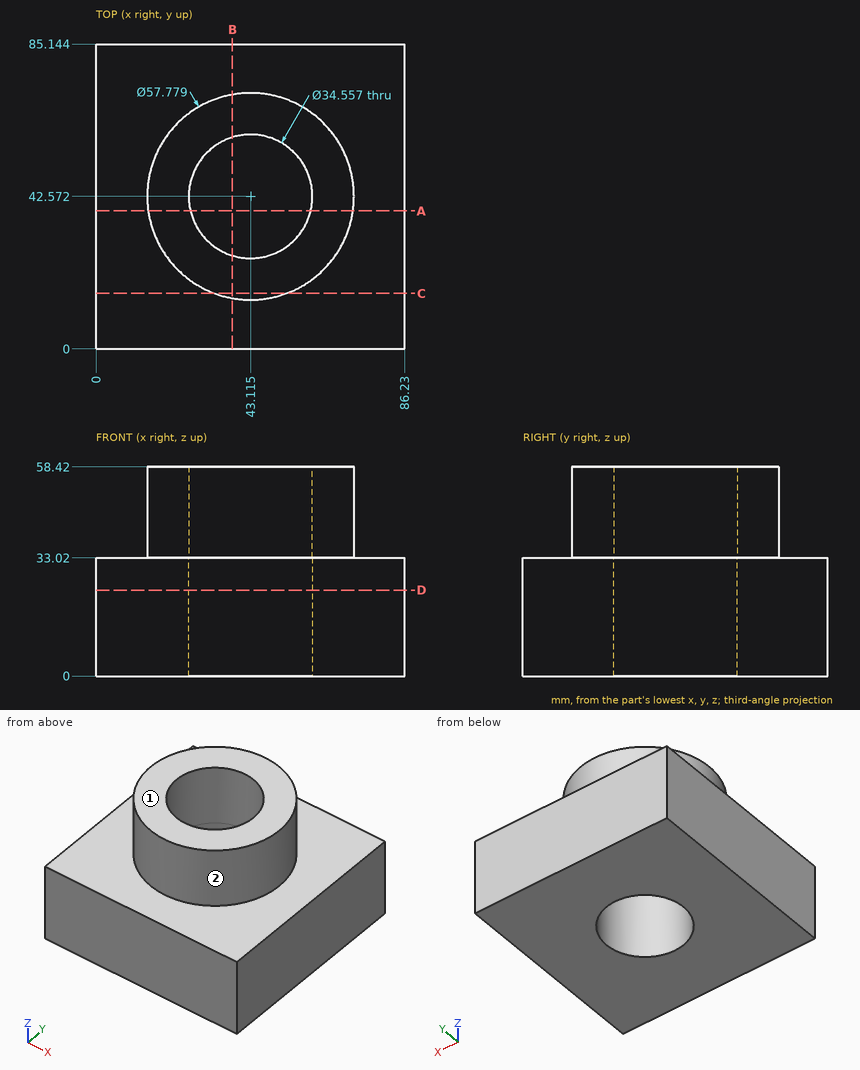
Geometry check sheet. Reference: drawing and pictorial views, mm from the part's lowest x, y, z. A direction names the side the tool comes from. Coordinates: 2 decimals unless noted, no trailing zeros. Order: outer loops, then holes, each group sorted by start corner. A loop starts at its lowest first (then second) coordinate and runs counter-clockwise, first axis right, second up.
1. Sectioned sample at A-A, the plane y = 38.5. Record the cut outline in (x, z).
Results found:
outline: (0, 0) - (26.32, 0) - (26.32, 58.42) - (14.51, 58.42) - (14.51, 33.02) - (0, 33.02) - close; (59.91, 0) - (86.23, 0) - (86.23, 33.02) - (71.72, 33.02) - (71.72, 58.42) - (59.91, 58.42) - close
2. Sectioned sample at B-B, the plane x = 38. Record the cut outline in (y, z) (1 decimal).
Results found:
outline: (0, 0) - (26.1, 0) - (26.1, 58.4) - (14.1, 58.4) - (14.1, 33) - (0, 33) - close; (59.1, 0) - (85.1, 0) - (85.1, 33) - (71, 33) - (71, 58.4) - (59.1, 58.4) - close
3. Go/stop test with flat-tipped pins: pin 1 Ø1 at (x, y) = (64.5, 13) entering from +Z; pin 2 Ø20.5 at (x, y) = (43.12, 42.57) entering from -Z; pin 3 Ø6 at (x, z) = (45, 38) entering from -Y; pin 4 Ø10 at (x, z) = (15.5, 41.5) entering from +Y. Record where each tip stops, or that it passes through.
Results found:
pin 1: stops at z = 33.02
pin 2: passes through
pin 3: stops at y = 13.68
pin 4: stops at y = 60.55
4. Scan lines: line 1 (Z direction, x = 75.5, y = 72); line 2 (X direction, y = 34, z = 13.5); line 3 (X direction, y = 36.5, z = 10.5). Record each from-to range of solid material in increasing order.
Results found:
line 1: z = 0 to 33.02
line 2: x = 0 to 28.11, 58.12 to 86.23
line 3: x = 0 to 26.94, 59.29 to 86.23
5. Sectioned sample at D-D, the plane z = 24. Record the cut outline in (x, y) (1 decimal).
Results found:
outline: (0, 0) - (86.2, 0) - (86.2, 85.1) - (0, 85.1) - close; hole circle Ø34.6 at (43.1, 42.6)
6. Set-up check for the marked faces 1 and 2: record each of +Z, -Z, +X, -X, +Y, -Y from which the full face is reachable in a straight line by a thin tool's end or side.
Results found:
face 1: +Z, +X, -X, +Y, -Y
face 2: +Z
7. Sectioned sample at C-C, the plane y = 15.5. Record the cut outline in (x, z).
Results found:
outline: (0, 0) - (86.23, 0) - (86.23, 33.02) - (53.2, 33.02) - (53.2, 58.42) - (33.03, 58.42) - (33.03, 33.02) - (0, 33.02) - close
